Here's the drawing with two shaded views (mm, measured from the low corner). I have some questions. A direction names the side the tool comes from. Coordinates: 2 decimals unless noted, no trailing zeros. Loops run counter-clockwise (first coordinate to the right, second up) from the corner with the lowest first, then second, coordinate; pieces in that order, holes last. Notation, with made-up numbers: (-25.75, 57.25) - (-5.75, 57.25) arc R21 cw to (-5.75, 96.25) - close; hole circle Ø7 at (-23, 36.25). An arc over 180 degrees is marked (long way). Use a Markdown table: item, result.
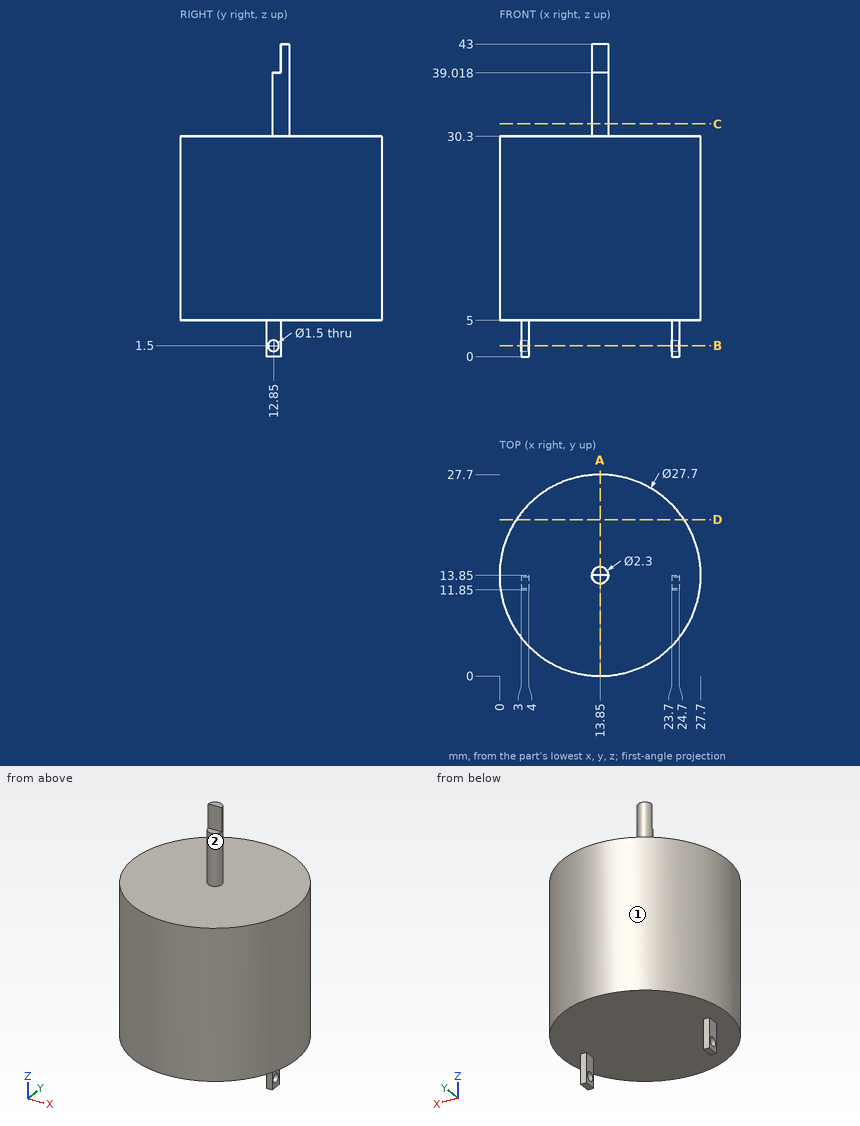
Q1. I want a section at A-A, the plane x = 13.85. Write out the boundary of the cut face in (y, z).
Check values:
| item | result |
|---|---|
| outline | (0, 5) - (27.7, 5) - (27.7, 30.3) - (15, 30.3) - (15, 43) - (13.85, 43) - (13.85, 39.02) - (12.7, 39.02) - (12.7, 30.3) - (0, 30.3) - close |
Q2. Will these pins go through, and if not, where does the flat tip stop? P1, Ø1.5, axis at x = 4.5, z = 24.5, coming from the +Y side; P2, Ø2, axis at y = 13, z = 3, coming from the -X side; P3, Ø1.6, axis at y = 13.5, z = 1.5, coming from the +X side.
Check values:
| item | result |
|---|---|
| P1 | y = 24.71 |
| P2 | x = 3 |
| P3 | x = 24.7 |
Q3. Please list where these lines run through material, in increasing order: L1, parallel to Z at x = 3.4, y = 12.85; L2, parallel to Z at x = 12.5, y = 25.25; L3, parallel to X at y = 5, z = 12.5 (1 decimal). Write a range as from..to.
Check values:
| item | result |
|---|---|
| L1 | 0..0.75, 2.25..30.3 |
| L2 | 5..30.3 |
| L3 | 3.2..24.5 |
Q4. I want a section at C-C, the plane z = 32. Write out the boundary of the cut face in (x, y).
Check values:
| item | result |
|---|---|
| outline | circle Ø2.3 at (13.85, 13.85) |
Q5. I want a section at B-B, the plane z = 1.5. Write out the boundary of the cut face in (x, y).
Check values:
| item | result |
|---|---|
| outline | (3, 11.85) - (4, 11.85) - (4, 12.1) - (3, 12.1) - close; (3, 13.6) - (4, 13.6) - (4, 13.85) - (3, 13.85) - close; (23.7, 11.85) - (24.7, 11.85) - (24.7, 12.1) - (23.7, 12.1) - close; (23.7, 13.6) - (24.7, 13.6) - (24.7, 13.85) - (23.7, 13.85) - close |
Q6. I want a section at D-D, the plane y = 21.5. Write out the boundary of the cut face in (x, z) (1 decimal), then the cut area to 3 significant figures.
Check values:
| item | result |
|---|---|
| outline | (2.3, 5) - (25.4, 5) - (25.4, 30.3) - (2.3, 30.3) - close |
| area | 584 mm^2 |
Q7. Which directions (+Z, -Z, +X, -X, +Y, -Y) give clear straight access to the entire face, cutting with the end or side of a thin tool? Please do the marked faces 1 and 2.
Check values:
| item | result |
|---|---|
| face 1 | +Z, -Z |
| face 2 | +Z |
